Here's how the part is built. I have some questions about the finished solid (model axes, mm). Face numbers are marked on the shaded views. A direction names the side the tool comes from. Give positions to 0.01 mm unless a question says otherwise; leave off trailing zeros. Loops run counter-clockwise (first coordinate to the right, second up) from the corner with the lowest first, then second, coordinate; pieces in that order, holes last. Notation, with made-up numbers: M 84,44.25 L 95,44.25 A7 ccw 95,49.25 Z; hole C -23,85.25 d2. An arc over 180 degrees is marked long. Write item = value, one per line. Start each with the question number.
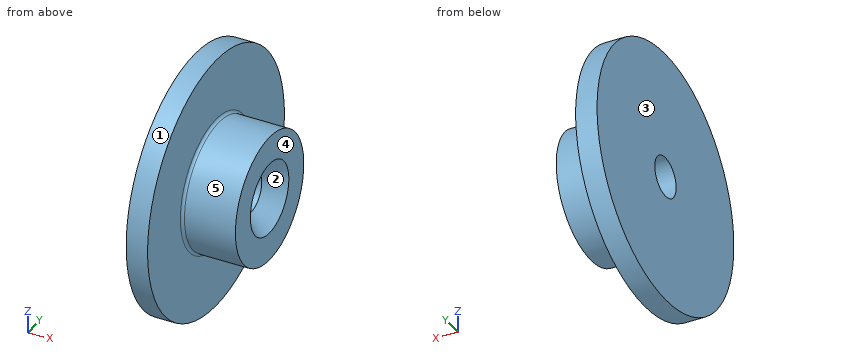
```python
from build123d import *

# Parameters (mm, degrees)
F2_R           = 0.79375
F4_D           = 11.90498
F4_CSINK_D     = 21.4376
F4_CSINK_ANGLE = 82


with BuildPart() as f1:
    # F0 (on Front) → F1 (revolve)
    with BuildSketch(Plane.XZ):
        Polygon((6.35, 38.1), (0, 38.1), (0, 0), (22.225, 0), (22.225, 19.05), (6.35, 19.05), align=None)
    revolve(axis=Axis((11.1125, 0, 0), (-1, 0, 0)))

    # F2
    f2_edges = [f1.edges().sort_by_distance(p)[0] for p in [
        (6.35, 0, -19.05),
    ]]
    fillet(f2_edges, radius=F2_R)

    # F4 (through all)
    with Locations(Plane.YZ.offset(22.225)):
        with Locations((0, 0)):
            CounterSinkHole(F4_D / 2, F4_CSINK_D / 2, counter_sink_angle=F4_CSINK_ANGLE)


solid = f1.part
```
Q1. If we section it at D-D, the plane y = 21: List the corners of the cut face in (x, z) for me, then the cut area to 3 significant figures.
Q2. We'd pull the mould along Z, two halves only. Please class the marked faces 1, 2 and 3: pulls with the +Z half, pulls with the -Z half, needs draft (parallel to the pull), parting line crosses it, or undercut.
Q3. On a 3-axis mill with a long thin cutter (end or side, diameter ignored), from which of +Z, -Z, +X, -X, +Y, -Y can I reach the whole of each face in a straight line? I mean the marked faces 4 and 5. Say none if no direction works.
Q4. Will these pins go through, and if not, where does the flat tip stop? pin 1 (12 mm diameter, centred on x = 9.5, z = -8.5, fed in from -Y); pin 2 (8 mm diameter, centred on x = 3, z = 1.5, fed in from +Y); pin 3 (4 mm diameter, centred on x = 5, z = -24.5, fed in from -Y); pin 4 (5 mm diameter, centred on x = 16, z = 22.5, fed in from +Y).
Q5. If we section it at C-C, the plane x = 15: List the corners of the cut face in (y, z) for me.
Q6. If I drill on line 1 along Y through (x, z) = (7, 0); line 2 along X through (y, z) = (28, 25.5); line 3 along Y through (x, z) = (5.25, -26), over which ranges is the centre line in solid material (lowest first)?
Resolved:
q1.outline = M 0,-31.79 L 6.35,-31.79 L 6.35,31.79 L 0,31.79 Z
q1.area = 404 mm²
q2.face_1 = parting line crosses it
q2.face_2 = undercut
q2.face_3 = needs draft
q3.face_4 = +Z, -Z, +X, +Y, -Y
q3.face_5 = +X
q4.pin_1 = -37.95
q4.pin_2 = 38.1
q4.pin_3 = -30.75
q4.pin_4 = through
q5.outline = C 0,0 d38.1; hole C 0,0 d11.9
q6.line_1 = -19.06 to -5.95, 5.95 to 19.06
q6.line_2 = 0 to 6.35
q6.line_3 = -27.85 to 27.85
